Verification items for the finished model (mm, model axes). Face numbers are marked on the shaded views. Coordinates: 2 decimals unless noted, no trailing zeros. Write each loop counter-clockwise with the first axis right and the second up, starting at its lowest first coordinate (ties: lowest second). Pieces come first, ordered by that corner, then holes. Notation, with made-up numbers: M 13,-21 L 51,-21 A20 cw 51,-13 Z; hole C 38.25,4.25 d7. An arc over 180 degrees is marked long. Answer in a Markdown table with one row per item.
from build123d import *

# Parameters (mm, degrees)
SKETCH_1_W             = 230
SKETCH_1_H             = 240
EXTRUDE_1_DEPTH        = 16
SKETCH_3_R             = 13
CUT_EXTRUDE_1_DEPTH    = 167.976046186
PATTERN_LINEAR_1_COUNT = 3
PATTERN_LINEAR_1_PITCH = 80
SKETCH_4_W             = 16
SKETCH_4_H             = 240
EXTRUDE_2_DEPTH        = 84
SKETCH_5_R             = 13
CUT_EXTRUDE_2_DEPTH    = 265.945277369
PATTERN_LINEAR_2_COUNT = 3
PATTERN_LINEAR_2_PITCH = 80


with BuildPart() as part:
    # 草图1 → 凸台-拉伸1 (new body)
    with BuildSketch(Plane.XY):
        Rectangle(SKETCH_1_W, SKETCH_1_H)
    extrude(amount=EXTRUDE_1_DEPTH)

    # 草图3 → 切除-拉伸1 (cut, through all)
    with BuildSketch(Plane.XY.offset(16)):
        with Locations((-73, 80)):
            Circle(SKETCH_3_R)
        with Locations((-14.5, 80)):
            Circle(SKETCH_3_R)
        with Locations((43.5, 80)):
            Circle(SKETCH_3_R)
    cut_extrude_1 = extrude(amount=-CUT_EXTRUDE_1_DEPTH, mode=Mode.SUBTRACT)

    # 阵列(线性)1: 切除-拉伸1 ×3
    with Locations(*[(0, -i * PATTERN_LINEAR_1_PITCH, 0) for i in range(1, PATTERN_LINEAR_1_COUNT)]):
        add(cut_extrude_1, mode=Mode.SUBTRACT)

    # 草图4 → 凸台-拉伸2 (add)
    with BuildSketch(Plane.XY.offset(16)):
        with Locations((107, 0)):
            Rectangle(SKETCH_4_W, SKETCH_4_H)
    extrude(amount=EXTRUDE_2_DEPTH)

    # 草图5 → 切除-拉伸2 (cut, through all)
    with BuildSketch(Plane.ZY.offset(-99)):
        with Locations((48, 80)):
            Circle(SKETCH_5_R)
    cut_extrude_2 = extrude(amount=-CUT_EXTRUDE_2_DEPTH, mode=Mode.SUBTRACT)

    # 阵列(线性)2: 切除-拉伸2 ×3
    with Locations(*[(0, -i * PATTERN_LINEAR_2_PITCH, 0) for i in range(1, PATTERN_LINEAR_2_COUNT)]):
        add(cut_extrude_2, mode=Mode.SUBTRACT)


solid = part.part
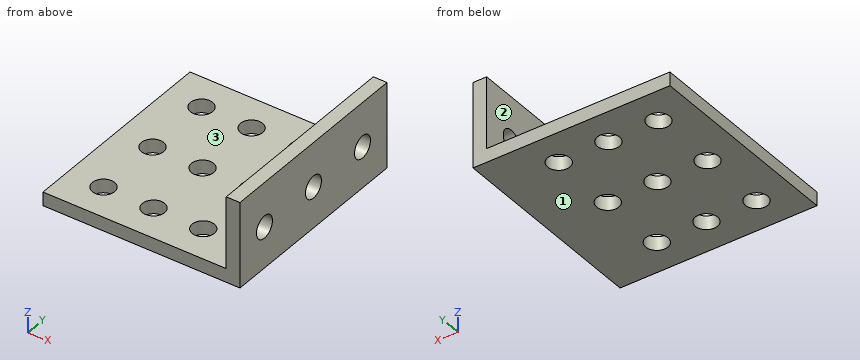
1) Depth check by flat-ended pin: pin 1 (1 mm diameter, centred on y = 80, z = 80.5, fed in from -X); pin 2 (8 mm diameter, centred on x = 9.5, y = 18, fed in from +Z). Enter the tip coordinate at first touch or a pass-through.
Response values:
| item | result |
|---|---|
| pin 1 | stops at x = 99 |
| pin 2 | stops at z = 16 |
2) Sectioned sample at C-C (x = -14.5). Record the cut outline in (y, z), then the cut area to 3 significant figures.
Response values:
| item | result |
|---|---|
| outline | M -120,0 L -93,0 L -93,16 L -120,16 Z; M -67,0 L -13,0 L -13,16 L -67,16 Z; M 13,0 L 67,0 L 67,16 L 13,16 Z; M 93,0 L 120,0 L 120,16 L 93,16 Z |
| area | 2,590 mm² |
3) Release check for a two-part mould opening along Z. For the marked faces 1, 2 and 3 record: +Z half, -Z half, draft (parallel to the pull), parting line (faces both ways), or undercut.
Response values:
| item | result |
|---|---|
| face 1 | -Z half |
| face 2 | draft |
| face 3 | +Z half |
4) Sectioned sample at A-A (z = 48). Record the cut outline in (x, y).
Response values:
| item | result |
|---|---|
| outline | M 99,-120 L 115,-120 L 115,-93 L 99,-93 Z; M 99,-67 L 115,-67 L 115,-13 L 99,-13 Z; M 99,13 L 115,13 L 115,67 L 99,67 Z; M 99,93 L 115,93 L 115,120 L 99,120 Z |
5) Sectioned sample at B-B (y = 80). Record the cut outline in (x, z), then the cut area to 3 significant figures.
Response values:
| item | result |
|---|---|
| outline | M -115,0 L -86,0 L -86,16 L -115,16 Z; M -60,0 L -27.5,0 L -27.5,16 L -60,16 Z; M -1.5,0 L 30.5,0 L 30.5,16 L -1.5,16 Z; M 56.5,0 L 115,0 L 115,35 L 99,35 L 99,16 L 56.5,16 Z; M 99,61 L 115,61 L 115,100 L 99,100 Z |
| area | 3,360 mm² |
6) Sectioned sample at D-D (y = -18.5). Record the cut outline in (x, z), then the cut area to 3 significant figures.
Response values:
| item | result |
|---|---|
| outline | M -115,0 L 115,0 L 115,100 L 99,100 L 99,16 L -115,16 Z |
| area | 5,020 mm² |
7) Thickness scan on L1, parallel to Y at x = 108.5, z = 48; L2, parallel to X at y = -90, z = 8; L3, parallel to X at y = -58.5, z = 87.5. Record the ranges inside material, lowest first. Write a range as [from, to].
Response values:
| item | result |
|---|---|
| L1 | y = [-120, -93], [-67, -13], [13, 67], [93, 120] |
| L2 | x = [-115, -81.31], [-64.69, -22.81], [-6.19, 35.19], [51.81, 115] |
| L3 | x = [99, 115] |
